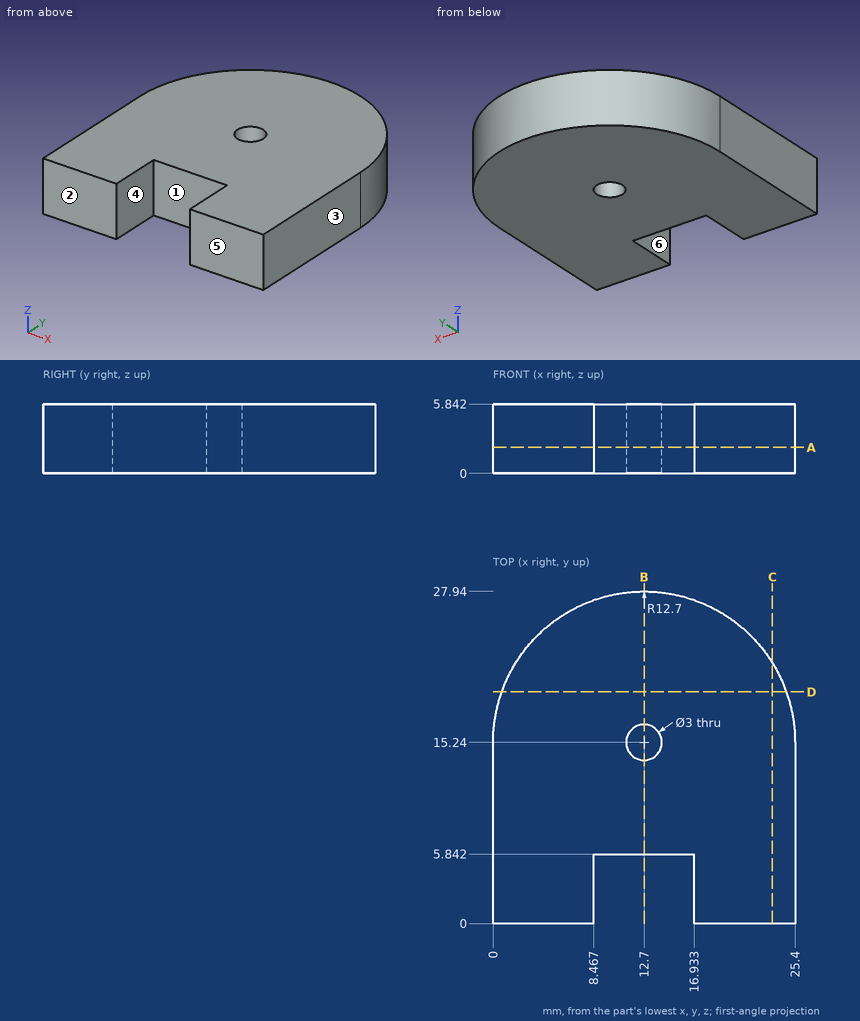
Input: dimensioned drawing with shaded views. Units: mm. Origin: part minimum x, y, z. A direction names the side the tool comes from. Coordinates: 2 decimals unless noted, no trailing zeros. Order: outer loops, then holes, each group sorted by start corner. A loop starts at its lowest first (then second) coordinate and runs counter-clockwise, first axis right, second up. Notation, with made-up numbers: M -33,-35.5 L -25,-35.5 A23 cw -25,-22.5 Z; hole C -17.5,-2.75 d8. An arc over 180 degrees is marked long. Write each question's results on one line, items separated by ' | '. Start each with the question number.
Item 1: Cut plane C-C (x = 23.5). Return loops of the section in (y, z), and give its area (3 significant figures).
Item 2: Cut plane B-B (x = 12.7). Return loops of the section in (y, z), and give its area (3 significant figures).
Item 3: First-contact query: pin 1 Ø1 at (x, z) = (3.5, 1.5) entering from +Y. Flat tip, straight axial feed; report the tip coordinate or a pass-through.
Item 4: Set-up query: the marked faces 5 and 6. Return all of +Z, -Z, +X, -X, +Y, -Y with unobstructed straight access to the full face (end or side cutting, diameter ignored); none if empty.
Item 5: Cut plane A-A (z = 2.2). Return loops of the section in (x, y).
Item 6: Line query: probe 1 along X at (y, z) = (5, 4.95); probe 2 along Y at (x, z) = (12.7, 3.05); probe 3 along Y at (x, z) = (13.75, 2.4) (1 decimal). Output: solid intervals per line, ascending.
Item 7: Cut plane D-D (y = 19.5). Return loops of the section in (x, z).
Item 8: Draft query along X for the marked faces 1, 2, 3 and 4. Return one class per face: pulls with the +X half, pulls with the -X half, needs draft (parallel to the pull), parting line crosses it, or undercut.
Checked values:
1) outline: M 0,0 L 21.92,0 L 21.92,5.84 L 0,5.84 Z | area: 128 mm2
2) outline: M 5.84,0 L 13.74,0 L 13.74,5.84 L 5.84,5.84 Z; M 16.74,0 L 27.94,0 L 27.94,5.84 L 16.74,5.84 Z | area: 112 mm2
3) pin 1: stops at y = 24.49
4) face 5: +Z, -Z, +X, -X, -Y | face 6: +Z, -Z, -Y
5) outline: M 0,0 L 8.47,0 L 8.47,5.84 L 16.93,5.84 L 16.93,0 L 25.4,0 L 25.4,15.24 A12.7 ccw 0,15.24 Z; hole C 12.7,15.24 d3
6) probe 1: x = 0 to 8.47, 16.93 to 25.4 | probe 2: y = 5.84 to 13.74, 16.74 to 27.94 | probe 3: y = 5.8 to 14.2, 16.3 to 27.9
7) outline: M 0.74,0 L 24.66,0 L 24.66,5.84 L 0.74,5.84 Z
8) face 1: undercut | face 2: needs draft | face 3: pulls with the +X half | face 4: undercut
